```python
from build123d import *

# Parameters (mm, degrees)
F1_DEPTH = 37.5
F2_DEPTH = 23
F4_DEPTH = 40
F7_DEPTH = 12.7279220614
F9_DEPTH = 123.6680763069


with BuildPart() as f1:
    # F0 (on Front) → F1 (new body, symmetric)
    with BuildSketch(Plane.XZ):
        Polygon((-40, -20), (0, -20), (0, -10), (-20, -10), (-20, 11.5470053838), (-69.2820323028, 40), (-74.2820323028, 31.3397459622), (-40, 11.5470053838), align=None)
        Polygon((-20, -10), (0, -10), (0, 0), (-20, 11.5470053838), align=None)
    extrude(amount=F1_DEPTH, both=True)

    # F0 (on Front) → F2 (cut, symmetric)
    with BuildSketch(Plane.XZ):
        Polygon((-20, -10), (0, -10), (0, 0), (-20, 11.5470053838), align=None)
    extrude(amount=F2_DEPTH, both=True, mode=Mode.SUBTRACT)

    # F3 (on Right) → F4 (join)
    with BuildSketch(Plane.YZ):
        Polygon((37.5, -20), (-37.5, -20), (-26, -40), (26, -40), align=None)
        Polygon((26, -40), (-26, -40), (-26, -58), (0, -58), (26, -58), align=None)
    extrude(amount=-F4_DEPTH)

    # F6 (on line) → F7 (join, through all)
    with BuildSketch(Plane(origin=(-20, 0, -20), x_dir=(0.7071067812, 0, -0.7071067812), z_dir=(0.7071067812, 0, 0.7071067812))):
        with BuildLine():
            Line((74.2842712475, 26), (28.2842712475, 26))
            Line((28.2842712475, 26), (28.2842712475, -26))
            Line((28.2842712475, -26), (74.2842712475, -26))
            ThreePointArc((74.2842712475, -26), (100.2842712475, 0), (74.2842712475, 26))
        make_face()
        Polygon((59.5618393831, 8.5), (74.2842712475, 17), (89.0067031118, 8.5), (89.0067031118, -8.5), (74.2842712475, -17), (59.5618393831, -8.5), align=None, mode=Mode.SUBTRACT)
    extrude(amount=-F7_DEPTH)

    # F8 (on face) → F9 (cut, through all)
    with BuildSketch(Plane(origin=(0, 0, 0), x_dir=(0.8660254038, 0, -0.5), z_dir=(0.5, 0, 0.8660254038))):
        with BuildLine():
            ThreePointArc((-53, -17), (-46, -24), (-39, -17))
            Line((-39, -17), (-39, 17))
            ThreePointArc((-39, 17), (-46, 24), (-53, 17))
            Line((-53, 17), (-53, 13))
            Line((-53, 13), (-61, 13))
            ThreePointArc((-61, 13), (-74, 0), (-61, -13))
            Line((-61, -13), (-53, -13))
            Line((-53, -13), (-53, -17))
        make_face()
    extrude(amount=-F9_DEPTH, mode=Mode.SUBTRACT)


solid = f1.part
```
Here's how the part is built. I have some questions about the finished solid (model axes, mm). A direction names the side the tool comes from. Give positions to 0.01 mm unless a question says otherwise; leave off trailing zeros. Order: outer loops, then holes, each group sorted by start corner. A loop starts at its lowest first (then second) coordinate and runs counter-clockwise, first axis right, second up. Notation, with made-up numbers: M 57,39.25 L 115,39.25 A16 cw 115,57.25 Z; hole C 11,19.5 d8. An arc over 180 degrees is marked long. Use a Markdown table: item, result. Add a question column.
1. Suppose I cut it at B-B (x = -9.5). List the corners of the cut face in (y, z) for me.
2. For pin 1 Ø5 at (x, z) = (-30, -26) entering from +Y; pin 2 Ø12 at (y, z) = (-22, -21.5) entering from +X; pin 3 Ø4 at (y, z) = (-12.5, -57.5) entering from +X, each with a flat end and sliding along its axis, tell me the tip position at first contact or that it passes through.
3. Suppose I cut it at D-D (z = -22). List the corners of the cut face in (x, y) for me.
4. On a 3-axis mill with a long thin cutter (end or side, diameter ignored), from which of +Z, -Z, +X, -X, +Y, -Y can I reach the whole of each face in a straight line? I mean faces 4 (the flat face through (38.5, 0.119, -87.374)), 5 (the flat face through (17.68, -0.119, -66.554)), 6 (the flat face through (0, -1, -20)), 7 (the flat face through (-40, -1, -23)), 8 (the cylindrical face through (-42, 24, 19)). Say none if no direction works.
5. Suppose I cut it at C-C (z = -68.5). List the corners of the cut face in (x, y) for me.
6. I need wall thicknesses on probe 1 along Y at (x, z) = (-18.5, -8.5); probe 2 along Z at (x, y) = (-8, -10.5); probe 3 along Y at (x, z) = (-49, 19.5). Which ranges of each line are inside material? Lowest first, please. Write a range as from..to.
7. Suppose I cut it at A-A (y = 5). List the corners of the cut face in (x, z) for me (3 decimals), and give its area (3 significant figures).
8. If we mould it in two halves opening along X, with no side actions, what happens to faces 1 (the flat face through (11, 0, -69)), 2 (the flat face through (33.37, -12.69, -82.24)), 3 (the flat face through (-10, 0, -10))? For each: +X half, -X half, draft (parallel to the pull), parting line (faces both ways), or undercut.
Results list:
| question | item | result |
|---|---|---|
| 1 | outline | M -37.5,-20 L -26,-40 L -26,-58 L 26,-58 L 26,-40 L 37.5,-20 L 37.5,5.48 L 23,5.48 L 23,-10 L -23,-10 L -23,5.48 L -37.5,5.48 Z |
| 2 | pin 1 | stops at y = 35.49 |
| 2 | pin 2 | stops at x = 0 |
| 2 | pin 3 | stops at x = 19.5 |
| 3 | outline | M -40,-36.35 L 0,-36.35 L 0,36.35 L -40,36.35 Z |
| 4 | face 4 | +Z, -X |
| 4 | face 5 | -Z, +X |
| 4 | face 6 | +Z, +X, +Y, -Y |
| 4 | face 7 | -Z, -X, +Y, -Y |
| 4 | face 8 | none |
| 5 | outline | M 10.5,-26 L 28.5,-26 L 28.5,-13.71 L 15.73,-8.5 L 15.73,8.5 L 28.5,13.71 L 28.5,26 L 10.5,26 Z |
| 6 | probe 1 | y = -37.5..-23, 23..37.5 |
| 6 | probe 2 | z = -58..-10 |
| 6 | probe 3 | y = -37.5..-20.28, 20.28..37.5 |
| 7 | outline | M -74.282,31.34 L -68.22,27.84 L -63.22,36.5 L -69.282,40 Z; M -40,-58 L 0,-58 L 13.117,-71.117 L 22.117,-62.117 L 0,-40 L 0,-10 L -20,-10 L -20,11.547 L -33.775,19.5 L -40,8.718 Z; M 33.937,-91.937 L 41.569,-99.569 L 50.569,-90.569 L 42.937,-82.937 Z |
| 7 | area | 2,950 mm² |
| 8 | face 1 | -X half |
| 8 | face 2 | undercut |
| 8 | face 3 | draft |
